Could you check a few things on this model? Use its own coordinates, in mm. Round coordinates to 2 decimals unless told otherwise and drop trailing zeros. Write each loop counter-clockwise with the first axis right and the second up, starting at its lowest first coordinate (ties: lowest second). Pieces come first, ordered by that corner, then holes. Notation, with made-up numbers: (87.25, 7) - (116.25, 7) arc R18 ccw to (116.25, 18) - close; hole circle Ø6 at (3, -29.5). An arc over 180 degrees is marked (long way). Write each question's results on one line, items separated by ' | '. Start each with the question number.
(1) Imagine slicing it at B-B on x = 0. State how many separate pieces and enclosed holes the cut face has, then the cut area to 3 significant figures.
(2) Imagine slicing it at A-A on y = 22.5. Write out the boundary of the cut face in (x, z).
(3) Please list where these lines run through material, in increasing order: line 1 (Y direction, x = -16, z = -1.95); line 2 (Y direction, x = 7.5, z = -3.1); line 3 (Y direction, x = 18.5, z = -1.45). Write a range as [from, to].
(4) Imagine slicing it at C-C on z = -2.35. Write out the boundary of the cut face in (x, y).
(5) Imagine slicing it at D-D on x = -17. Write out the boundary of the cut face in (y, z), then the cut area to 3 significant figures.
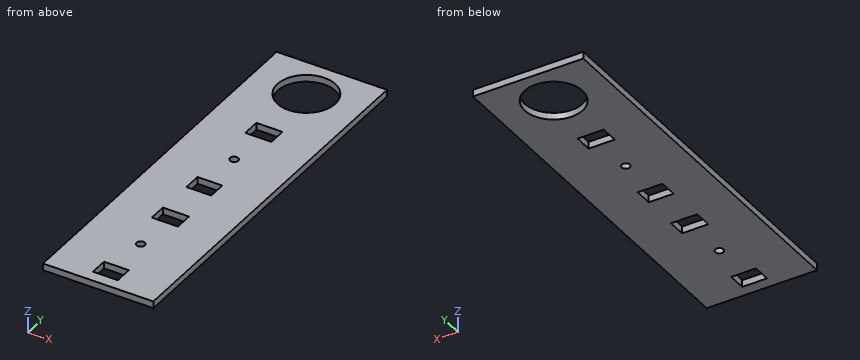
```python
from build123d import *

# Parameters (mm, degrees)
ESQUISSE1_W             = 80
ESQUISSE1_H             = 275
BOSS_EXTRU_1_DEPTH      = 5
ESQUISSE2_R             = 21
ESQUISSE2_R_2           = 3
ESQUISSE2_W             = 18
ESQUISSE2_H             = 13
ESQUISSE2_W_2           = 19
ENL_V_MAT_EXTRU_1_DEPTH = 6


with BuildPart() as part:
    # Esquisse1 → Boss.-Extru.1 (new body)
    with BuildSketch(Plane.XY):
        Rectangle(ESQUISSE1_W, ESQUISSE1_H)
    extrude(amount=-BOSS_EXTRU_1_DEPTH)

    # Esquisse2 → Enlèv. mat.-Extru.1 (cut, through all)
    with BuildSketch(Plane.XY):
        with Locations((0, 107.5)):
            Circle(ESQUISSE2_R)
        with Locations((0, 22.5)):
            Circle(ESQUISSE2_R_2)
        with Locations((0, -87.5)):
            Circle(ESQUISSE2_R_2)
        with Locations((0, -122.5)):
            Rectangle(ESQUISSE2_W, ESQUISSE2_H)
        with Locations((0, 57.5)):
            Rectangle(ESQUISSE2_W_2, ESQUISSE2_H)
        with Locations((0, -12.5)):
            Rectangle(ESQUISSE2_W, ESQUISSE2_H)
        with Locations((0, -52.5)):
            Rectangle(ESQUISSE2_W_2, ESQUISSE2_H)
    extrude(amount=-ENL_V_MAT_EXTRU_1_DEPTH, mode=Mode.SUBTRACT)


solid = part.part
```
Response:
1) separate pieces: 8 | enclosed holes: 0 | area: 845 mm²
2) outline: (-40, -5) - (-3, -5) - (-3, 0) - (-40, 0) - close; (3, -5) - (40, -5) - (40, 0) - (3, 0) - close
3) line 1: [-137.5, 93.9], [121.1, 137.5] | line 2: [-137.5, -129], [-116, -59], [-46, -19], [-6, 51], [64, 87.88], [127.12, 137.5] | line 3: [-137.5, 97.56], [117.44, 137.5]
4) outline: (-40, -137.5) - (40, -137.5) - (40, 137.5) - (-40, 137.5) - close; hole circle Ø42 at (0, 107.5); hole (-9.5, -59) - (9.5, -59) - (9.5, -46) - (-9.5, -46) - close; hole (-9.5, 51) - (9.5, 51) - (9.5, 64) - (-9.5, 64) - close; hole (-9, -129) - (9, -129) - (9, -116) - (-9, -116) - close; hole (-9, -19) - (9, -19) - (9, -6) - (-9, -6) - close; hole circle Ø6 at (0, -87.5); hole circle Ø6 at (0, 22.5)
5) outline: (-137.5, -5) - (95.17, -5) - (95.17, 0) - (-137.5, 0) - close; (119.83, -5) - (137.5, -5) - (137.5, 0) - (119.83, 0) - close | area: 1,250 mm²
